Part model, mm, in its own coordinate system. Round coordinates to 2 decimals unless told otherwise and drop trailing zeros. Loops run counter-clockwise (first coordinate to the right, second up) from the corner with the lowest first, then second, coordinate; pieces in that order, holes last. Notation, with made-up numbers: (-8, 44) - (34, 44) arc R11 ccw to (34, 61) - close; hole circle Ø6 at (-37, -27.5). An arc over 180 degrees is marked (long way). Put each result on its own line as item: value.
from build123d import *

# Parameters (mm, degrees)
SKETCH_1_R      = 3
SKETCH_1_R_2    = 1.5
EXTRUDE_1_DEPTH = 2


with BuildPart() as part:
    # 草图1 → 凸台-拉伸1 (new body)
    with BuildSketch(Plane.XY):
        with BuildLine():
            Line((23.59477523, -43.872599913), (43.741142958, -56.320462917))
            Line((43.741142958, -56.320462917), (43.741142958, -68.872599913))
            Line((43.741142958, -68.872599913), (15.241142958, -68.872599913))
            Line((15.241142958, -68.872599913), (-13.258857042, -68.872599913))
            Line((-13.258857042, -68.872599913), (-13.258857042, -56.320462917))
            Line((-13.258857042, -56.320462917), (6.887510685, -43.872599913))
            ThreePointArc((6.887510685, -43.872599913), (15.241142958, -35.51896764), (23.59477523, -43.872599913))
        make_face()
        with Locations((15.241142958, -61.872599913)):
            Circle(SKETCH_1_R, mode=Mode.SUBTRACT)
        with Locations((40.241142958, -61.872599913)):
            Circle(SKETCH_1_R_2, mode=Mode.SUBTRACT)
        with Locations(Location((-9.758857042, -61.872599913, 0), (0, 0, 180))):
            Circle(SKETCH_1_R_2, mode=Mode.SUBTRACT)
        with Locations((15.241142958, -43.872599913)):
            Circle(SKETCH_1_R, mode=Mode.SUBTRACT)
    extrude(amount=EXTRUDE_1_DEPTH)


solid = part.part
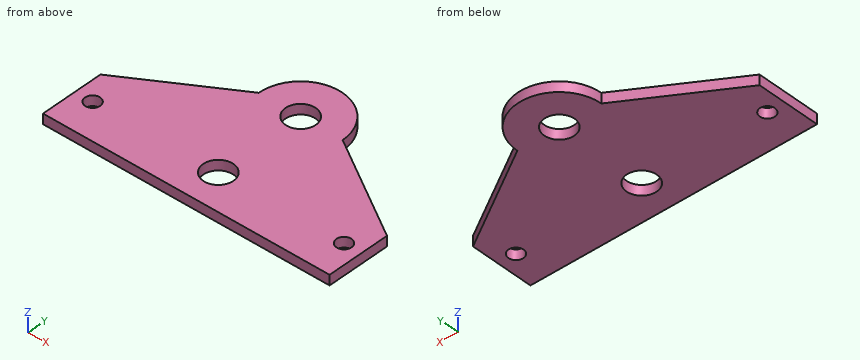
1. Band-saw the part on D-D (y = -53.5). List the corners of the cut face in (x, z), plus the area to 3 significant figures.
A:
outline: (-8.69, 0) - (39.18, 0) - (39.18, 2) - (-8.69, 2) - close
area: 95.7 mm²
2. Pin check, flat tips, straight feed: P1, Ø3.5, axis at x = -9.76, y = -61.87, coming from the -Z side; P2, Ø1, axis at y = -42, z = 1, coming from the -X side; P3, Ø5, axis at x = 15.24, y = -43.87, coming from the -Z side. Stop position of each tip, or through.
A:
P1: stops at z = 0
P2: stops at x = 7
P3: passes through
3. Band-saw the part on A-A (y = -42.5). List the corners of the cut face in (x, z).
A:
outline: (7, 0) - (12.57, 0) - (12.57, 2) - (7, 2) - close; (17.91, 0) - (23.48, 0) - (23.48, 2) - (17.91, 2) - close
4. Band-saw the part on B-B (z = 0.9). List the corners of the cut face in (x, y), plus the area to 3 significant figures.
A:
outline: (-13.26, -68.87) - (43.74, -68.87) - (43.74, -56.32) - (23.59, -43.87) arc R8.35 ccw to (6.89, -43.87) - (-13.26, -56.32) - close; hole circle Ø3 at (-9.76, -61.87); hole circle Ø6 at (15.24, -61.87); hole circle Ø6 at (15.24, -43.87); hole circle Ø3 at (40.24, -61.87)
area: 1,210 mm²
5. Band-saw the part on C-C (x = 34.5). List the corners of the cut face in (y, z), plus the area to 3 significant figures.
A:
outline: (-68.87, 0) - (-50.61, 0) - (-50.61, 2) - (-68.87, 2) - close
area: 36.5 mm²
6. Probe line 1 along X through (y, z) = (-62.5, 1.5); line 2 along X through (y, z) = (-44, 0.25); line 3 along X through (y, z) = (-64, 1). List the from-to ranges inside material, lowest first. Write a range as [from, to].
A:
line 1: x = [-13.26, -11.12], [-8.4, 12.31], [18.17, 38.88], [41.6, 43.74]
line 2: x = [6.68, 12.24], [18.24, 23.8]
line 3: x = [-13.26, 13.13], [17.36, 43.74]
